from build123d import *

# Parameters (mm, degrees)
F0_W     = 101.6
F0_H     = 101.6
F1_DEPTH = 101.6
F2_R     = 25.4
F3_DEPTH = 101.6
F6_W     = 50.8
F6_H     = 50.8
F7_DEPTH = 101.6
F8_R     = 6.35
F9_R     = 5.08


with BuildPart() as f1:
    # F0 (on Top) → F1 (new body)
    with BuildSketch(Plane.XY):
        Rectangle(F0_W, F0_H)
    extrude(amount=F1_DEPTH)

    # F2 (on face) → F3 (join)
    with BuildSketch(Plane.XY.offset(101.6)):
        Circle(F2_R)
    extrude(amount=F3_DEPTH)

    # F4 (on face) → F5 (revolve)
    with BuildSketch(Plane.XY.offset(203.2)):
        with BuildLine():
            Line((0, -25.4), (0, -38.1))
            ThreePointArc((0, -38.1), (38.1, 0), (0, 38.1))
            Line((0, 38.1), (0, 25.4))
            ThreePointArc((0, 25.4), (17.9605122421, 17.9605122421), (25.4, 0))
            ThreePointArc((25.4, 0), (17.9605122421, -17.9605122421), (0, -25.4))
        make_face()
        with BuildLine():
            Line((0, 25.4), (0, -25.4))
            ThreePointArc((0, -25.4), (17.9605122421, -17.9605122421), (25.4, 0))
            ThreePointArc((25.4, 0), (17.9605122421, 17.9605122421), (0, 25.4))
        make_face()
    revolve(axis=Axis((0, 0, 203.2), (0, -1, 0)))

    # F6 (on face) → F7 (cut)
    with BuildSketch(Plane.XZ.offset(50.8)):
        with Locations((0, 50.8)):
            Rectangle(F6_W, F6_H)
    extrude(amount=-F7_DEPTH, mode=Mode.SUBTRACT)

    # F8
    f8_edges = [f1.edges().sort_by_distance(p)[0] for p in [
        (50.8, 0, 101.6),
        (0, -50.8, 101.6),
        (-50.8, 0, 101.6),
        (0, 50.8, 101.6),
        (50.8, 0, 0),
        (50.8, 50.8, 50.8),
        (50.8, -50.8, 50.8),
        (-50.8, -50.8, 50.8),
        (0, -50.8, 0),
        (-50.8, 0, 0),
        (0, 50.8, 0),
        (-50.8, 50.8, 50.8),
    ]]
    fillet(f8_edges, radius=F8_R)

    # F9
    f9_edges = [f1.edges().sort_by_distance(p)[0] for p in [
        (-25.4, 0, 101.6),
    ]]
    fillet(f9_edges, radius=F9_R)


solid = f1.part
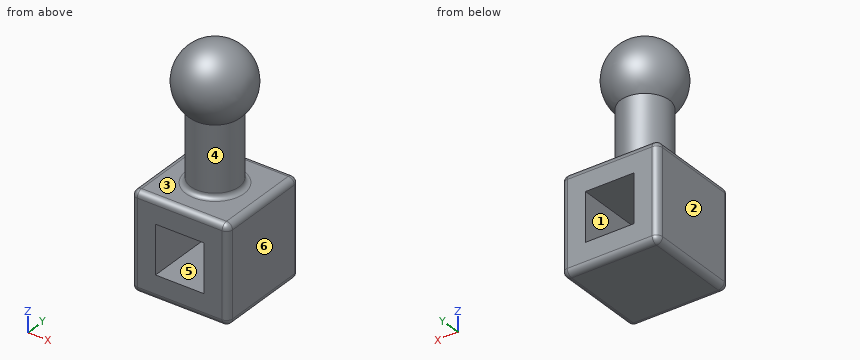
Source: CAD feature listing. Evaluate the final solid. Frame: model axes, mm. Face numbers are marked on the shaded views. A direction names the side the tool comes from. Give positions to 0.01 mm unless a question says otherwise; leave off trailing zeros. Write each loop counter-clockwise with the first axis right and the second up, starting at its lowest first coordinate (ties: lowest second). Pieces come first, ordered by that corner, then holes. Notation, with made-up numbers: M 39,-26 L 61,-26 A32 cw 61,9 Z; hole C 9,12.25 d1. An arc over 180 degrees is marked long. Return JSON: item names as keys, results as strings. Group by question number.
1) Pull-direction query (X, two-part tool) for the marked faces 3, 4, 5 and 6; classes: pulls with the +X half, pulls with the -X half, needs draft (parallel to the pull), parting line crosses it, or undercut.
2) Material intervals for line 1 along X through (y, z) = (17.5, 26.5); line 2 along Z through (x, y) = (31.5, 12.5); line 3 along Z through (x, y) = (-34, 34), sorted ascending. Write a range as [from, to].
3) Cut plane D-D, the plane z = 150. Output: boundary loops of the cut face in (x, y), plus the area to 3 significant figures.
4) Cut plane A-A, the plane x = 0. Output: boundary loops of the cut face in (y, z).
5) Set-up query: the marked faces 1 and 2. Return all of +Z, -Z, +X, -X, +Y, -Y with unobstructed straight access to the full face (end or side cutting, diameter ignored); none if empty.
6) Cut plane B-B, the plane y = -35. Output: boundary loops of the cut face in (x, z), plus the area to 3 significant figures.
7) Cut plane C-C, the plane y = 0. Output: boundary loops of the cut face in (x, z).
8) Pin query (flat end, axial travel): P1, Ø6, axis at y = -23, z = 118.5, coming from the -X side; P2, Ø12, axis at x = -2, y = -6, coming from the +Z side; P3, Ø12, axis at x = -37.5, z = 200, coming from the +Y side. Return the tip coordinate at first contact, or that it passes through.
Recorded:
{
 "1": {"face 3": "needs draft", "face 4": "parting line crosses it", "face 5": "undercut", "face 6": "pulls with the +X half"},
 "2": {"line 1": "x = [-50.8, -25.4], [25.4, 50.8]", "line 2": "z = [0, 101.6], [185.79, 220.61]", "line 3": "z = [0, 101.6]"},
 "3": {"outline": "C 0,0 d50.8", "area": "2,030 mm²"},
 "4": {"outline": "M -50.8,6.35 A6.35 ccw -44.45,0 L 44.45,0 A6.35 ccw 50.8,6.35 L 50.8,25.4 L -50.8,25.4 Z; M -50.8,76.2 L 50.8,76.2 L 50.8,95.25 A6.35 ccw 44.45,101.6 L 30.48,101.6 A5.08 cw 25.4,106.68 L 25.4,174.8 A38.1 ccw long -25.4,174.8 L -25.4,106.68 A5.08 cw -30.48,101.6 L -44.45,101.6 A6.35 ccw -50.8,95.25 Z"},
 "5": {"face 1": "+Y, -Y", "face 2": "+Z, -Z, -X, +Y, -Y"},
 "6": {"outline": "M -50.8,6.35 A6.35 ccw -44.45,0 L 44.45,0 A6.35 ccw 50.8,6.35 L 50.8,95.25 A6.35 ccw 44.45,101.6 L -44.45,101.6 A6.35 ccw -50.8,95.25 Z; C 0,203.2 d30.11; hole M -25.4,25.4 L 25.4,25.4 L 25.4,76.2 L -25.4,76.2 Z", "area": "8,420 mm²"},
 "7": {"outline": "M -50.8,6.35 A6.35 ccw -44.45,0 L 44.45,0 A6.35 ccw 50.8,6.35 L 50.8,95.25 A6.35 ccw 44.45,101.6 L 30.48,101.6 A5.08 cw 25.4,106.68 L 25.4,174.8 A38.1 ccw long -25.4,174.8 L -25.4,106.68 A5.08 cw -30.48,101.6 L -44.45,101.6 A6.35 ccw -50.8,95.25 Z; hole M -25.4,25.4 L 25.4,25.4 L 25.4,76.2 L -25.4,76.2 Z"},
 "8": {"P1": "stops at x = -15.66", "P2": "stops at z = 241.3", "P3": "stops at y = 21.23"}
}
